Study the drawing (mm; zero at the part's minimum x, y, z) and answer. A direction names the side the tool comes from. Give positions to 0.01 mm unless a question says otherwise; leave off trailing zeros. Order: outer loops, then holes, each group sorted by start corner. A loop starts at its lowest first (then second) coordinate and runs counter-clockwise, first axis right, second up. Notation, with made-up numbers: (26.25, -29) -> (78.25, -29) arc R35 cw to (78.25, 6) -> close; hole circle Ø11 at (67.5, 3). An arc over 180 degrees is marked (long way). One line per question, with ' | ' between items. Start each with the question number.
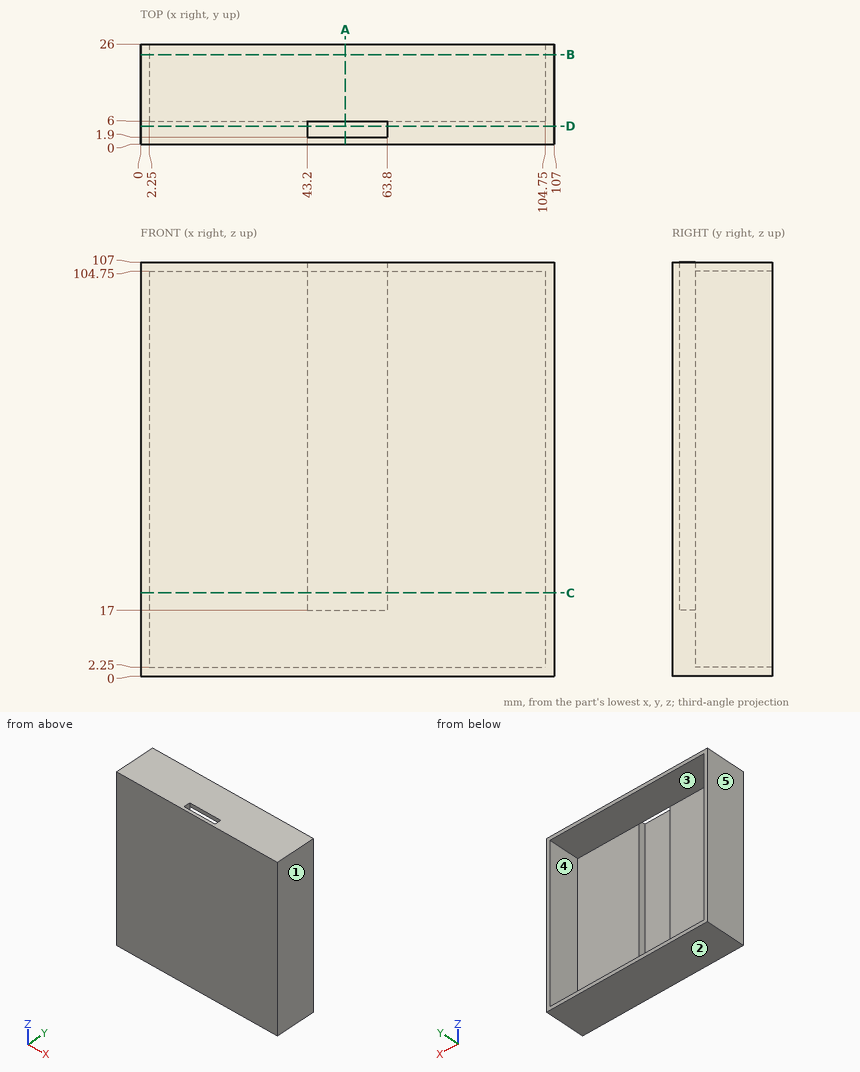
Q1. A cutting plane is placed at C-C, the plane z = 21.5. Determine the outline of the cut face in (x, y).
Q2. A cutting plane is placed at B-B, the plane y = 23.25. Determine the outline of the cut face in (x, z), then the cut area to 3 significant figures.
Q3. A cutting plane is placed at A-A, the plane x = 53. Determine the outline of the cut face in (y, z), then the cut area to 3 significant figures.
Q4. Find the intervals of material crossed by line 1 (X direction, y = 21.5, z = 33.5); line 2 (X direction, y = 3.25, z = 102), in increasing order.
Q5. Determine the mould class of the marked faces 1, 2 and 3 for opening direction X: pulls with the +X half, pulls with the -X half, needs draft (parallel to the pull), parting line crosses it, or undercut.
Q6. Which of the six approach directions +Z, -Z, +X, -X, +Y, -Y give full straight-line access (tool end or side, diameter ignored) to the marked faces 4 and 5?
Q7. A cutting plane is placed at D-D, the plane y = 4.75. Determine the outline of the cut face in (x, z).
Q8. Given P1, Ø10, axis at x = 23, z = 73.5, coming from the +Y side; P2, Ø10.5, axis at x = 50.5, z = 51.5, coming from the +Y side, each flat-ended and moving along its own axis, determine where each tip first touches the part or whether it passes through.
Geometry results:
1) outline: (0, 0) -> (107, 0) -> (107, 26) -> (104.75, 26) -> (104.75, 6) -> (63.8, 6) -> (63.8, 1.9) -> (43.2, 1.9) -> (43.2, 6) -> (2.25, 6) -> (2.25, 26) -> (0, 26) -> close
2) outline: (0, 0) -> (107, 0) -> (107, 107) -> (0, 107) -> close; hole (2.25, 2.25) -> (104.75, 2.25) -> (104.75, 104.75) -> (2.25, 104.75) -> close | area: 943 mm²
3) outline: (0, 0) -> (26, 0) -> (26, 2.25) -> (6, 2.25) -> (6, 17) -> (1.9, 17) -> (1.9, 107) -> (0, 107) -> close; (6, 104.75) -> (26, 104.75) -> (26, 107) -> (6, 107) -> close | area: 363 mm²
4) line 1: 0 to 2.25, 104.75 to 107 | line 2: 0 to 43.2, 63.8 to 107
5) face 1: pulls with the +X half | face 2: needs draft | face 3: undercut
6) face 4: +Y | face 5: +Z, -Z, -X, +Y, -Y
7) outline: (0, 0) -> (107, 0) -> (107, 107) -> (63.8, 107) -> (63.8, 17) -> (43.2, 17) -> (43.2, 107) -> (0, 107) -> close
8) P1: y = 6 | P2: y = 1.9
